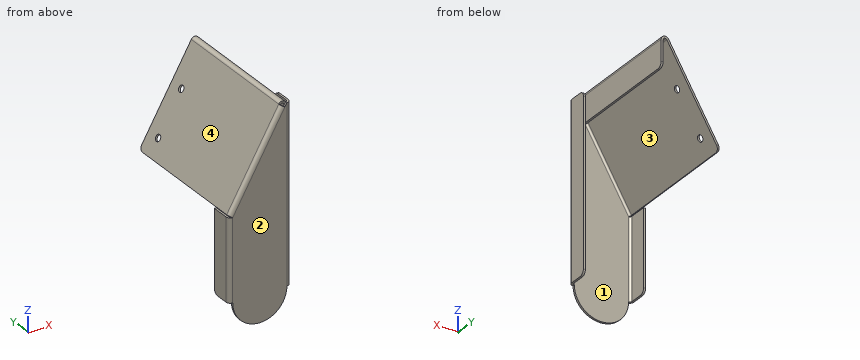
from build123d import *

# Parameters (mm, degrees)
BOSS_EXTRUDE1_DEPTH     = 2
BOSS_EXTRUDE3_DEPTH     = 2
EDGE_FLANGE1_DEPTH      = 81.3
EDGE_FLANGE1_BEND_DEPTH = 174.830743609
EDGE_FLANGE2_DEPTH      = 103.8
EDGE_FLANGE3_DEPTH      = 134
M6_CLEARANCE_HOLE1_D    = 6.6
FILLET1_R               = 5


# Sheet-metal steps are written as plain solids
with BuildPart() as part:
    # Sketch1 → Boss-Extrude1 (new body)
    with BuildSketch(Plane(origin=(0, 0, 0), x_dir=(1, 0, 0), z_dir=(0, 1, 0))):
        with BuildLine():
            Line((-27, -108.3), (-27, -27))
            ThreePointArc((-27, -27), (-19.091883092, -7.908116908), (0, 0))
            Line((0, 0), (0, -108.3))
            Line((0, -108.3), (-27, -108.3))
        make_face()
    boss_extrude1 = extrude(amount=BOSS_EXTRUDE1_DEPTH)

    # Mirror1: Boss-Extrude1 across plane
    add(boss_extrude1.mirror(Plane(origin=(0, 0, 0), x_dir=(0, 0, 1), z_dir=(1, 0, 0))))

    # Sketch15 → Boss-Extrude3 (add)
    with BuildSketch(Plane(origin=(0, 2, 0), x_dir=(1, 0, 0), z_dir=(0, 1, 0))):
        Polygon((-27, -108.3), (27, -201.830743609), (27, -108.3), align=None)
    extrude(amount=-BOSS_EXTRUDE3_DEPTH)

    # Edge-Flange1 section (across the edge) → Edge-Flange1 (add)
    with BuildSketch(Plane(origin=(-29, 2, 27), x_dir=(1, 0, 0), z_dir=(0, 0, 1))):
        with BuildLine():
            Line((-2, 2), (-2, 20))
            Line((-2, 20), (0, 20))
            Line((0, 20), (0, 2))
            ThreePointArc((0, 2), (0.585786438, 0.585786438), (2, 0))
            Line((2, 0), (2, -2))
            ThreePointArc((2, -2), (-0.828427125, -0.828427125), (-2, 2))
        make_face()
    extrude(amount=EDGE_FLANGE1_DEPTH)

    # Edge-Flange1 section 2 (across the edge) → Edge-Flange1 bend (add)
    with BuildSketch(Plane(origin=(29, 2, 201.830743609), x_dir=(-1, 0, 0), z_dir=(0, 0, -1))):
        with BuildLine():
            Line((-2, 2), (-2, 20))
            Line((-2, 20), (0, 20))
            Line((0, 20), (0, 2))
            ThreePointArc((0, 2), (0.585786438, 0.585786438), (2, 0))
            Line((2, 0), (2, -2))
            ThreePointArc((2, -2), (-0.828427125, -0.828427125), (-2, 2))
        make_face()
    extrude(amount=EDGE_FLANGE1_BEND_DEPTH)

    # Edge-Flange2 section (across the edge) → Edge-Flange2 (add)
    with BuildSketch(Plane(origin=(-28.732050808, 2, 109.3), x_dir=(0.8660254037844362, 3.491481338843134e-15, -0.5000000000000044), z_dir=(0.5000000000000044, 0, 0.8660254037844362))):
        with BuildLine():
            Line((-2, 2), (-2, 136))
            Line((-2, 136), (0, 136))
            Line((0, 136), (0, 2))
            ThreePointArc((0, 2), (0.585786438, 0.585786438), (2, 0))
            Line((2, 0), (2, -2))
            ThreePointArc((2, -2), (-0.828427125, -0.828427125), (-2, 2))
        make_face()
    extrude(amount=EDGE_FLANGE2_DEPTH)

    # Edge-Flange3 section (across the edge) → Edge-Flange3 (add)
    with BuildSketch(Plane(origin=(26.9, 138, 205.657538528), x_dir=(-1, 0, 0), z_dir=(0, -1, 0))):
        with BuildLine():
            Line((-2, 7.464101615), (-2, 33.464101615))
            Line((-2, 33.464101615), (0, 33.464101615))
            Line((0, 33.464101615), (0, 7.464101615))
            ThreePointArc((0, 7.464101615), (1.48236191, 5.532249963), (3.732050808, 6.464101615))
            Line((3.732050808, 6.464101615), (5.464101615, 5.464101615))
            ThreePointArc((5.464101615, 5.464101615), (0.96472382, 3.60039831), (-2, 7.464101615))
        make_face()
    extrude(amount=EDGE_FLANGE3_DEPTH)

    # M6 Clearance Hole1 (through all)
    with Locations(Plane(origin=(-68.877326422, 0, 39.766342951), x_dir=(-0.5000000000000046, -2.00195274507357e-15, -0.8660254037844362), z_dir=(0.8660254037844362, 3.4674838688193673e-15, -0.5000000000000046))):
        with Locations((-144.573890731, 123), (-98.29055123, 123)):
            Hole(M6_CLEARANCE_HOLE1_D / 2)

    # Fillet1
    fillet1_edges = [part.edges().sort_by_distance(p)[0] for p in [
        (-30, 22, 27),
        (30, 22, 201.830743609),
        (30, 22, 27),
        (-29.598076211, 138, 109.8),
        (27.9, 138, 172.193436913),
    ]]
    fillet(fillet1_edges, radius=FILLET1_R)


solid = part.part
Model file for the job. Use its own axes, mm. Face numbers are marked on the shaded views. Round coordinates to 2 decimals unless told otherwise and drop trailing zeros. Order: outer loops, then holes, each group sorted by start corner. A loop starts at its lowest first (then second) coordinate and runs counter-clockwise, first axis right, second up.
(1) Pin check, flat tips, straight feed: pin 1 (4.5 mm diameter, centred on x = -28.5, y = 8.5, fed in from +Z); pin 2 (8 mm diameter, centred on y = 101, z = 182, fed in from +X); pin 3 (1.6 mm diameter, centred on x = -30, z = 52, fed in from +Y); pin 4 (6 mm diameter, centred on x = -11.5, z = 153, fed in from -Y). Stop position of each tip, or through.
(2) Drill centre lines: line 1 (Y direction, x = -5, z = 137); line 2 (X direction, y = 16.5, z = 138); line 3 (Z direction, x = 12.5, y = 64). Where is each one in solid material? Low to high.
(3) Band-saw the part on B-B (z = 89.5). List the corners of the cut face in (x, y).
(4) Band-saw the part on A-A (y = 9.5). List the corners of the cut face in (x, z), then the cut area to 3 significant figures.
(5) Band-saw the part on C-C (y = 129). List the corners of the cut face in (x, z), then the cut area to 3 significant figures.
(6) Band-saw the part on D-D (z = 22). List the corners of the cut face in (x, y), then the cut area to 3 significant figures.
(7) Pull direction X, two halves, no side cores. Call the marked faces 1, 2, 3 and 4: released by +X, released by -X, zero draft, split by the parting line, or undercut.
Verdict:
1. pin 1: stops at z = 117.6
1. pin 2: stops at x = 28.9
1. pin 3: stops at y = 22
1. pin 4: passes through
2. line 1: y = 0 to 2
2. line 2: x = -14.47 to -12.16, 29 to 31
2. line 3: z = 180.72 to 184.72
3. outline: (-31, 4) arc R4 ccw to (-27, 0) - (27, 0) arc R4 ccw to (31, 4) - (31, 22) - (29, 22) - (29, 4) arc R2 cw to (27, 2) - (-27, 2) arc R2 cw to (-29, 4) - (-29, 22) - (-31, 22) - close
4. outline: (-31, 27) - (-29, 27) - (-29, 108.3) - (-31, 108.3) - close; (-30.46, 110.3) - (-28.73, 109.3) - (23.17, 199.19) arc R2 cw to (26.9, 198.19) - (26.9, 172.19) - (28.9, 172.19) - (28.9, 198.19) arc R4 ccw to (21.44, 200.19) - close; (29, 27) - (31, 27) - (31, 201.83) - (29, 201.83) - close
4. area: 788 mm2
5. outline: (-30.46, 110.3) - (-28.73, 109.3) - (23.17, 199.19) arc R2 cw to (26.9, 198.19) - (26.9, 172.19) - (28.9, 172.19) - (28.9, 198.19) arc R4 ccw to (21.44, 200.19) - close
5. area: 275 mm2
6. outline: (-26.53, 0) - (26.53, 0) - (26.53, 2) - (-26.53, 2) - close
6. area: 106 mm2
7. face 1: undercut
7. face 2: zero draft
7. face 3: undercut
7. face 4: released by -X
